```python
from build123d import *

# Parameters (mm, degrees)
F1_DEPTH = 6.35
F2_DEPTH = 914.4


with BuildPart() as f1:
    # F0 (on Top) → F1 (new body)
    with BuildSketch(Plane.XY):
        with BuildLine():
            ThreePointArc((-10.16, -4.4064424835), (-9.2585377355, 6.0763323116), (0, 11.0744))
            Line((0, 11.0744), (0, 26.3144))
            Line((0, 26.3144), (-10.16, 26.3144))
            ThreePointArc((-10.16, 26.3144), (-13.4590659426, 7.9300363387), (-28.4382271537, -3.227624381))
            Line((-28.4382271537, -3.227624381), (-23.3582271537, -12.0264424835))
            Line((-23.3582271537, -12.0264424835), (-10.16, -4.4064424835))
        make_face()
        with BuildLine():
            ThreePointArc((10.148152514, -4.4336594269), (10.8403652051, -2.2646892899), (11.0744, 0))
            ThreePointArc((11.0744, 0), (7.8307833376, 7.8307833376), (0, 11.0744))
            ThreePointArc((0, 11.0744), (-9.2585377355, 6.0763323116), (-10.16, -4.4064424835))
            ThreePointArc((-10.16, -4.4064424835), (-0.0148418743, -11.0743900545), (10.148152514, -4.4336594269))
        make_face()
        with BuildLine():
            ThreePointArc((0, 11.0744), (7.8307833376, 7.8307833376), (11.0744, 0))
            ThreePointArc((11.0744, 0), (10.8403652051, -2.2646892899), (10.148152514, -4.4336594269))
            Line((10.148152514, -4.4336594269), (23.3463796676, -12.0536594269))
            Line((23.3463796676, -12.0536594269), (28.4263796676, -3.2548413244))
            ThreePointArc((28.4263796676, -3.2548413244), (13.4364974773, 7.9131265949), (10.148152514, 26.3144))
            Line((10.148152514, 26.3144), (0, 26.3144))
            Line((0, 26.3144), (0, 11.0744))
        make_face()
        with BuildLine():
            Line((23.3463796676, -12.0536594269), (10.148152514, -4.4336594269))
            ThreePointArc((10.148152514, -4.4336594269), (-0.0148418743, -11.0743900545), (-10.16, -4.4064424835))
            Line((-10.16, -4.4064424835), (-23.3582271537, -12.0264424835))
            Line((-23.3582271537, -12.0264424835), (-18.2782271537, -20.8252605859))
            ThreePointArc((-18.2782271537, -20.8252605859), (-0.0001467991, -13.082077915), (18.2663796676, -20.8524775293))
            Line((18.2663796676, -20.8524775293), (23.3463796676, -12.0536594269))
        make_face()
    extrude(amount=F1_DEPTH)

    # F0 (on Top) → F2 (cut)
    with BuildSketch(Plane.XY):
        with BuildLine():
            ThreePointArc((10.148152514, -4.4336594269), (10.8403652051, -2.2646892899), (11.0744, 0))
            ThreePointArc((11.0744, 0), (7.8307833376, 7.8307833376), (0, 11.0744))
            ThreePointArc((0, 11.0744), (-9.2585377355, 6.0763323116), (-10.16, -4.4064424835))
            ThreePointArc((-10.16, -4.4064424835), (-0.0148418743, -11.0743900545), (10.148152514, -4.4336594269))
        make_face()
    extrude(amount=F2_DEPTH, mode=Mode.SUBTRACT)


solid = f1.part
```
Verification items for the finished model (mm, model axes). Round coordinates to 2 decimals unless told otherwise and drop trailing zeros. Loops run counter-clockwise (first coordinate to the right, second up) from the corner with the lowest first, then second, coordinate; pieces in that order, holes last. Notation, with made-up numbers: (55, 48.5) -> (92, 48.5) arc R16 ccw to (92, 74.5) -> close; hole circle Ø1 at (-31, -34). An arc over 180 degrees is marked (long way). Answer as a JSON object with one key per item and string values.
Q1. Go/stop test with flat-tipped pins: P1, Ø1, axis at x = -17.5, z = 2.5, coming from the +Y side; P2, Ø2, axis at y = 12.5, z = 5, coming from the -X side; P3, Ø1.5, axis at y = -0.5, z = 3.5, coming from the +X side. Record where each tip stops, or that it passes through.
Data:
{"P1": "stops at y = 3.43", "P2": "stops at x = -11.62", "P3": "stops at x = 23.29"}
Q2. Scan lines: line 1 (X direction, y = -17, z = 3.75); line 2 (X direction, y = 10, z = 6.25); line 3 (Y direction, x = -5.5, z = 6). Record each from-to range of solid material in increasing order. Write a range as from..to.
Data:
{"line 1": "x = -20.49..-13.57, 13.53..20.49", "line 2": "x = -12.31..-4.76, 4.76..12.28", "line 3": "y = -13.68..-9.61, 9.61..26.31"}
Q3. Section check A-A (x = -1). Record the boundary of the cut face in (y, z), then the cut area to 3 significant figures.
Data:
{"outline": "(-13.1, 0) -> (-11.03, 0) -> (-11.03, 6.35) -> (-13.1, 6.35) -> close; (11.03, 0) -> (26.31, 0) -> (26.31, 6.35) -> (11.03, 6.35) -> close", "area": "110 mm2"}
Q4. Draft check along Y on faces 1 (the flat face through (12, -2, 6.35)), 2 (the cylindrical face through (13.579, 7.686, 3.131)), 3 (the flat face through (0, 26.314, 3)). Enter one of: pulls with the +Y half, pulls with the -Y half, needs draft (parallel to the pull), parting line crosses it, or undercut.
Data:
{"face 1": "needs draft", "face 2": "undercut", "face 3": "pulls with the +Y half"}
Q5. Section check C-C (z = 2.25). Record the boundary of the cut face in (x, y).
Data:
{"outline": "(-28.44, -3.23) -> (-18.28, -20.83) arc R25.4 cw to (18.27, -20.85) -> (28.43, -3.25) arc R25.4 cw to (10.15, 26.31) -> (-10.16, 26.31) arc R25.4 cw to start; hole circle Ø22.15 at (0, 0)"}
Q6. Section check D-D (x = 22.5). Record the boundary of the cut face in (y, z), then the cut area to 3 significant figures.
Data:
{"outline": "(-13.52, 0) -> (-0.82, 0) -> (-0.82, 6.35) -> (-13.52, 6.35) -> close", "area": "80.6 mm2"}
Q7. Section check B-B (y = -5.5). Record the boundary of the cut face in (x, z), then the cut area to 3 significant figures.
Data:
{"outline": "(-27.13, 0) -> (-9.61, 0) -> (-9.61, 6.35) -> (-27.13, 6.35) -> close; (9.61, 0) -> (27.13, 0) -> (27.13, 6.35) -> (9.61, 6.35) -> close", "area": "222 mm2"}
